Build history of the part. All positions in model axes, mm. Coordinates: 2 decimals unless noted, no trailing zeros. Loops run counter-clockwise (first coordinate to the right, second up) from the corner with the lowest first, then second, coordinate; pieces in that order, holes last. Notation, with made-up numbers: M 44,7 L 94,7 A18 cw 94,38 Z; hole C 80.5,30.5 d10. An arc over 180 degrees is marked long. Write each question's results on one line, items separated by ' | '. Start each with the question number.
from build123d import *

# Parameters (mm, degrees)
SKETCH1_W           = 1150
SKETCH1_H           = 545
SKETCH1_R           = 87.5
BOSS_EXTRUDE1_DEPTH = 10


with BuildPart() as part:
    # Sketch1 → Boss-Extrude1 (new body)
    with BuildSketch(Plane.XY):
        with Locations((-65, 0)):
            Rectangle(SKETCH1_W, SKETCH1_H)
        with Locations((-300, 0)):
            Circle(SKETCH1_R, mode=Mode.SUBTRACT)
        Circle(SKETCH1_R, mode=Mode.SUBTRACT)
        with Locations((300, 0)):
            Circle(SKETCH1_R, mode=Mode.SUBTRACT)
    extrude(amount=BOSS_EXTRUDE1_DEPTH)


solid = part.part
1. Wall check: line 1 along X through (y, z) = (-4.5, 6.5); line 2 along Y through (x, z) = (-300, 8.25); line 3 along X through (y, z) = (-27.5, 6.75). Give the ranges that are in metal, low to high.
2. Mould opens along X. For faces 1 (the flat face through (-73, -57, 10)), 2 (the cylindrical face through (-64.49, 59.14, 4.93)) say: +X half, -X half, draft (parallel to the pull), parting line (faces both ways), or undercut.
3. Band-saw the part on B-B, the plane y = 0. List the corners of the cut face in (x, z), plus the area to 3 significant figures.
4. Band-saw the part on D-D, the plane x = 246.5. List the corners of the cut face in (y, z).
5. Band-saw the part on A-A, the plane x = 0. List the corners of the cut face in (y, z), plus the area to 3 significant figures.
6. Band-saw the part on C-C, the plane z = 8.5. List the corners of the cut face in (x, y).
Checked values:
1) line 1: -640 to -387.38, -212.62 to -87.38, 87.38 to 212.62, 387.38 to 510 | line 2: -272.5 to -87.5, 87.5 to 272.5 | line 3: -640 to -383.07, -216.93 to -83.07, 83.07 to 216.93, 383.07 to 510
2) face 1: draft | face 2: undercut
3) outline: M -640,0 L -387.5,0 L -387.5,10 L -640,10 Z; M -212.5,0 L -87.5,0 L -87.5,10 L -212.5,10 Z; M 87.5,0 L 212.5,0 L 212.5,10 L 87.5,10 Z; M 387.5,0 L 510,0 L 510,10 L 387.5,10 Z | area: 6,250 mm²
4) outline: M -272.5,0 L -69.24,0 L -69.24,10 L -272.5,10 Z; M 69.24,0 L 272.5,0 L 272.5,10 L 69.24,10 Z
5) outline: M -272.5,0 L -87.5,0 L -87.5,10 L -272.5,10 Z; M 87.5,0 L 272.5,0 L 272.5,10 L 87.5,10 Z | area: 3,700 mm²
6) outline: M -640,-272.5 L 510,-272.5 L 510,272.5 L -640,272.5 Z; hole C -300,0 d175; hole C 0,0 d175; hole C 300,0 d175
